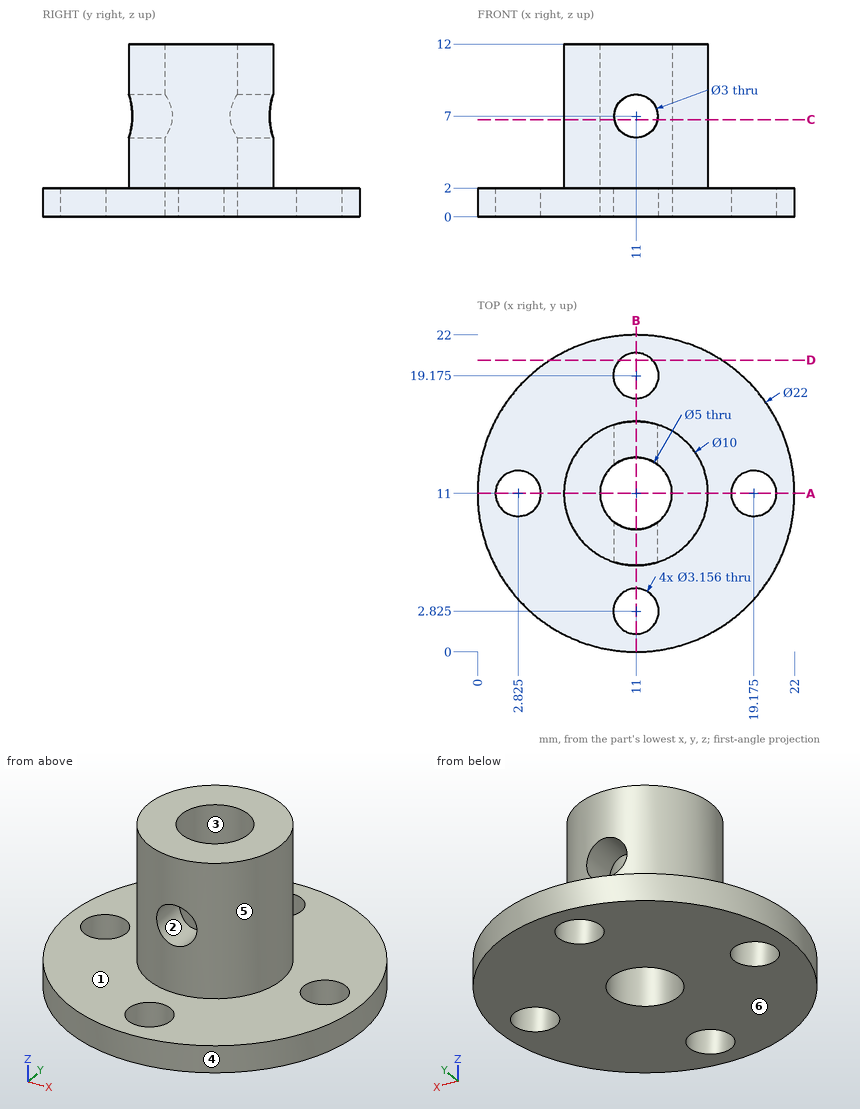
Verification items for this drawing (mm, ordinates from the low corner). A direction names the side the tool comes from. Coordinates: 2 decimals unless noted, no trailing zeros. Write each loop counter-clockwise with the first axis right and the second up, starting at its lowest first coordinate (ties: lowest second). Pieces come first, ordered by that corner, then holes. Notation, with made-up numbers: M 30.25,86 L 61.25,86 A23 cw 61.25,120 Z; hole C 87.5,58 d6. An arc over 180 degrees is marked long. One line per item, written item: value. Start each with the question number.
(1) Scan lines: line 1 along Y through (x, z) = (11, 0.9); line 2 along Y through (x, z) = (11, 3); line 3 along Z through (x, y) = (11, 6.75). Record each from-to range of solid material in increasing order. Write a range as [from, to].
(2) Sectioned sample at A-A, the plane y = 11. Enter the section's corners in (x, z).
(3) Sectioned sample at B-B, the plane x = 11. Enter the section's corners in (y, z), and give its area (3 significant figures).
(4) Sectioned sample at D-D, the plane y = 20.25. Enter the section's corners in (x, z) (1 decimal).
(5) Tool access check on the marked faces 5 and 6. Record the directions out of +Z, -Z, +X, -X, +Y, -Y that give a thin tool (end or side, any length) a straight path to the whole face; none if there is none.
(6) Sectioned sample at C-C, the plane z = 6.75. Enter the section's corners in (x, y).
(7) Depth check by flat-ended pin: pin 1 (4 mm diameter, centred on x = 11, y = 2.825, fed in from +Z); pin 2 (1.5 mm diameter, centred on y = 6.5, z = 10.5, fed in from +X); pin 3 (3.5 mm diameter, centred on x = 11, z = 7, fed in from +Y). Enter the tip coordinate at first touch or a pass-through.
(8) Release check for a two-part mould opening along X. For the marked faces 1, 2, 3 and 4 record: released by +X, released by -X, zero draft, split by the parting line, or undercut.
Filled sheet:
1. line 1: [0, 1.25], [4.4, 8.5], [13.5, 17.6], [20.75, 22]
1. line 2: [6, 8.5], [13.5, 16]
1. line 3: [0, 5.5], [8.5, 12]
2. outline: M 0,0 L 1.25,0 L 1.25,2 L 0,2 Z; M 4.4,0 L 8.5,0 L 8.5,12 L 6,12 L 6,2 L 4.4,2 Z; M 13.5,0 L 17.6,0 L 17.6,2 L 16,2 L 16,12 L 13.5,12 Z; M 20.75,0 L 22,0 L 22,2 L 20.75,2 Z
3. outline: M 0,0 L 1.25,0 L 1.25,2 L 0,2 Z; M 4.4,0 L 8.5,0 L 8.5,5.5 L 6,5.5 L 6,2 L 4.4,2 Z; M 6,8.5 L 8.5,8.5 L 8.5,12 L 6,12 Z; M 13.5,0 L 17.6,0 L 17.6,2 L 16,2 L 16,5.5 L 13.5,5.5 Z; M 13.5,8.5 L 16,8.5 L 16,12 L 13.5,12 Z; M 20.75,0 L 22,0 L 22,2 L 20.75,2 Z
3. area: 56.4 mm²
4. outline: M 5,0 L 9.8,0 L 9.8,2 L 5,2 Z; M 12.2,0 L 17,0 L 17,2 L 12.2,2 Z
5. face 5: +Z
5. face 6: -Z, +X, -X, +Y, -Y
6. outline: M 9.52,6.22 L 9.52,8.98 A2.5 cw 9.52,13.02 L 9.52,15.78 A5 ccw Z; M 12.48,6.22 A5 ccw 12.48,15.78 L 12.48,13.02 A2.5 cw 12.48,8.98 Z
7. pin 1: z = 2
7. pin 2: x = 14.31
7. pin 3: y = 16
8. face 1: zero draft
8. face 2: undercut
8. face 3: undercut
8. face 4: split by the parting line
